Part model, mm, in its own coordinate system. Face numbers are marked on the shaded views. A direction names the side the tool comes from. Coordinates: 2 decimals unless noted, no trailing zeros. Loops run counter-clockwise (first coordinate to the right, second up) from the corner with the lowest first, then second, coordinate; pieces in that order, holes last. Notation, with made-up numbers: M 51,-38.75 L 89,-38.75 A26 ccw 89,-7.75 Z; hole C -38,62.25 d4. An arc over 180 degrees is marked long. Use a Markdown table: item, result. Add a question column.
1) Band-saw the part on B-B (z = 0). List the corners of the cut face in (x, y), plus the area to 3 significant figures.
2) Band-saw the part on D-D (y = 0.5). List the corners of the cut face in (x, z), plus the area to 3 significant figures.
3) Tool access for the marked faces 1, 2, 3, 4 and 5: list every direction of +Z, -Z, +X, -X, +Y, -Y with a clear straight run to the whole face (end or side of a thin tool).
4) Band-saw the part on A-A (y = 5). List the corners of the cut face in (x, z), plus the area to 3 significant figures.
5) Pin check, flat tips, straight feed: pin 1 Ø1.4 at (x, z) = (6.5, 6.5) entering from -Y; pin 2 Ø1.5 at (y, z) = (8.5, 0) entering from +X; pin 3 Ø5 at (x, y) = (10.5, 20.5) entering from +Z; pin 4 Ø3 at (y, z) = (1, 0) entering from +X. Stop position of each tip, or through.
6) Pull direction X, two halves, no side cores. Call the marked faces 6, 7 and 8: released by +X, released by -X, zero draft, split by the parting line, or undercut.
7) Wall check: probe 1 along X at (y, z) = (8, 2.75); probe 2 along Y at (x, z) = (6.5, 2.75); probe 3 along Z at (x, y) = (1.35, 0). Give the ranges that are in metal, low to high. Write a range as from..to.
8) Band-saw the part on C-C (x = 5). List the corners of the cut face in (y, z).
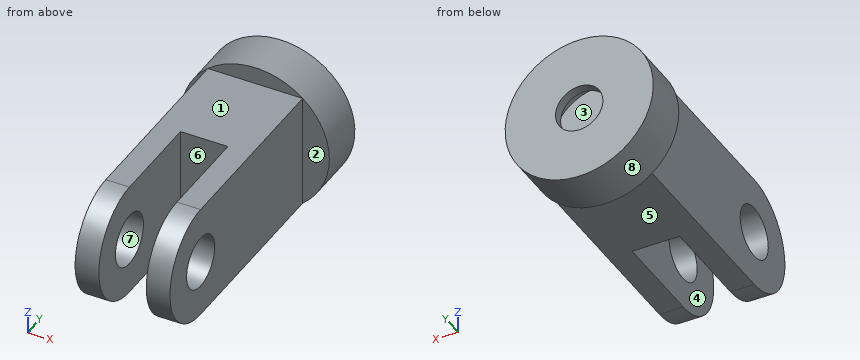
from build123d import *

# Parameters (mm, degrees)
SKETCH1_R           = 2.75
BOSS_EXTRUDE1_DEPTH = 10
SKETCH3_R           = 7.810249676
BOSS_EXTRUDE3_DEPTH = 5
SKETCH4_R           = 5
CUT_EXTRUDE1_DEPTH  = 4
SKETCH5_R           = 6.128825336
SKETCH5_R_2         = 2.5
BOSS_EXTRUDE4_DEPTH = 1
SKETCH7_W           = 20.888038085
SKETCH7_H           = 5
CUT_EXTRUDE2_DEPTH  = 13


with BuildPart() as part:
    # Sketch1 → Boss-Extrude1 (new body)
    with BuildSketch(Plane.YZ):
        with BuildLine():
            Line((0, 6), (20, 6))
            Line((20, 6), (20, -6))
            Line((20, -6), (0, -6))
            ThreePointArc((0, -6), (-6, 0), (0, 6))
        make_face()
        with Locations(Location((0, 0, 0), (0, 0, 270))):
            Circle(SKETCH1_R, mode=Mode.SUBTRACT)
    extrude(amount=BOSS_EXTRUDE1_DEPTH)

    # Sketch3 → Boss-Extrude3 (add)
    with BuildSketch(Plane(origin=(0, 20, 0), x_dir=(-1, 0, 0), z_dir=(0, 1, 0))):
        with Locations(Location((-5, 0, 0), (0, 0, 230.194428908))):
            Circle(SKETCH3_R)
    extrude(amount=BOSS_EXTRUDE3_DEPTH)

    # Sketch4 → Cut-Extrude1 (cut)
    with BuildSketch(Plane(origin=(0, 25, 0), x_dir=(-1, 0, 0), z_dir=(0, 1, 0))):
        with Locations(Location((-5, 0, 0), (0, 0, 90))):
            Circle(SKETCH4_R)
    extrude(amount=-CUT_EXTRUDE1_DEPTH, mode=Mode.SUBTRACT)

    # Sketch5 → Boss-Extrude4 (add)
    with BuildSketch(Plane(origin=(0, 25, 0), x_dir=(-1, 0, 0), z_dir=(0, 1, 0))):
        with Locations((-5, 0)):
            Circle(SKETCH5_R)
        with Locations(Location((-5, 0, 0), (0, 0, 90))):
            Circle(SKETCH5_R_2, mode=Mode.SUBTRACT)
    extrude(amount=-BOSS_EXTRUDE4_DEPTH)

    # Sketch7 → Cut-Extrude2 (cut, symmetric)
    with BuildSketch(Plane(origin=(0, 0, 0), x_dir=(0, 1, 0), z_dir=(0, 0, 1))):
        with Locations((-0.444019042, -5)):
            Rectangle(SKETCH7_W, SKETCH7_H)
    extrude(amount=CUT_EXTRUDE2_DEPTH, both=True, mode=Mode.SUBTRACT)


solid = part.part
Entries:
| question | item | result |
|---|---|---|
| 1 | outline | M -2.81,20 L 0,20 L 0,2.75 L 2.5,2.75 L 2.5,10 L 7.5,10 L 7.5,2.75 L 10,2.75 L 10,20 L 12.81,20 L 12.81,25 L 7.5,25 L 7.5,24 L 10,24 L 10,21 L 0,21 L 0,24 L 2.5,24 L 2.5,25 L -2.81,25 Z; M 0,-6 L 2.5,-6 L 2.5,-2.75 L 0,-2.75 Z; M 7.5,-6 L 10,-6 L 10,-2.75 L 7.5,-2.75 Z |
| 1 | area | 196 mm2 |
| 2 | outline | M 0,-6 L 2.5,-6 L 2.5,-2.7 L 0,-2.7 Z; M 0,2.7 L 2.5,2.7 L 2.5,6 L 0,6 Z; M 7.5,-6 L 10,-6 L 10,-2.7 L 7.5,-2.7 Z; M 7.5,2.7 L 10,2.7 L 10,6 L 7.5,6 Z |
| 2 | area | 33.0 mm2 |
| 3 | face 1 | +Z, +X, -X, -Y |
| 3 | face 2 | +Z, -Z, +X, -Y |
| 3 | face 3 | none |
| 3 | face 4 | +Z, -Z, -Y |
| 3 | face 5 | -Z, +X, -X, -Y |
| 4 | outline | M 0,-6 L 2.5,-6 L 2.5,6 L 0,6 Z; M 7.5,-6 L 10,-6 L 10,6 L 7.5,6 Z |
| 4 | area | 60.0 mm2 |
| 5 | pin 1 | y = 10 |
| 5 | pin 2 | x = 10 |
| 5 | pin 3 | z = 7.21 |
| 5 | pin 4 | through |
| 6 | face 6 | undercut |
| 6 | face 7 | zero draft |
| 6 | face 8 | split by the parting line |
| 7 | probe 1 | 0..2.5, 7.5..10 |
| 7 | probe 2 | 10..21, 24..25 |
| 7 | probe 3 | -6..-2.75, 2.75..6 |
| 8 | outline | M 10,-6 L 20,-6 L 20,-7.81 L 25,-7.81 L 25,-2.5 L 24,-2.5 L 24,-5 L 21,-5 L 21,5 L 24,5 L 24,2.5 L 25,2.5 L 25,7.81 L 20,7.81 L 20,6 L 10,6 Z |
